Verification items for the finished model (mm, model axes). Coordinates: 2 decimals unless noted, no trailing zeros. Order: outer loops, then holes, each group sorted by start corner. A loop starts at its lowest first (then second) coordinate and runs counter-clockwise, first axis right, second up. Notation, with made-up numbers: (73, -9) -> (124, -9) arc R18 cw to (124, 25) -> close; hole circle Ø11 at (-34, -38). An arc over 180 degrees is marked (long way). Write each question's results on one line, items separated by ' | '. Start each with the question number.
(1) Cross-section at B-B on z = 5.5. Enter the section's corners in (x, y), and give its area (3 significant figures).
(2) Cross-section at C-C on x = 1.25. Enter the section's corners in (y, z), and give its area (3 significant figures).
(3) Cross-section at A-A on x = 4.75. Enter the section's corners in (y, z), and give its area (3 significant figures).
(4) Go/stop test with flat-tipped pins: pin 1 (12 mm diameter, centred on x = 9, z = 21, fed in from +Y); pin 2 (2 mm diameter, centred on x = 3, y = 7, fed in from -Z); pin 3 (2.5 mm diameter, centred on y = -2, z = 7.5, fed in from +X); pin 4 (1 mm diameter, centred on x = -9, z = 14.5, fed in from -Y). Record where each tip stops, or that it passes through.
(5) Thickness scan on probe 1 along X at (y, z) = (-4, 22.25); probe 2 along Y at (x, z) = (2.5, 23); probe 3 along X at (y, z) = (-3.25, 8). Record the ranges inside material, lowest first. Write a range as [from, to].
(6) Cross-section at D-D on y = -12. Enter the section's corners in (x, z).
(7) Draft check along Y on faces 1 (the flat face through (-0.2, -6.5, 0)), 2 (the flat face through (-4, 0, 12)). Enter one of: +Y half, -Y half, draft (parallel to the pull), parting line (faces both ways), or undercut.
```python
from build123d import *

# Parameters (mm, degrees)
BOSS_EXTRU_1_DEPTH = 25


with BuildPart() as part:
    # Esquisse2 → Boss.-Extru.1 (new body)
    with BuildSketch(Plane.XY):
        with BuildLine():
            ThreePointArc((-4, 4.472135955), (-2.140932539, 5.605034154), (0, 6))
            Line((0, 6), (0, 15))
            ThreePointArc((0, 15), (-2.018355219, 14.863587797), (-4, 14.456832295))
            Line((-4, 14.456832295), (-4, 4.472135955))
        make_face()
        with BuildLine():
            Line((0, 15), (0, 6))
            ThreePointArc((0, 6), (4.242640687, 4.242640687), (6, 0))
            ThreePointArc((6, 0), (2.449489743, -5.477225575), (-4, -4.472135955))
            Line((-4, -4.472135955), (-4, -14.456832295))
            ThreePointArc((-4, -14.456832295), (9.082951062, -11.937336386), (15, 0))
            ThreePointArc((15, 0), (10.606601718, 10.606601718), (0, 15))
        make_face()
        with BuildLine():
            ThreePointArc((-4, -4.472135955), (-6, 0), (-4, 4.472135955))
            Line((-4, 4.472135955), (-4, 14.456832295))
            ThreePointArc((-4, 14.456832295), (-15, 0), (-4, -14.456832295))
            Line((-4, -14.456832295), (-4, -4.472135955))
        make_face()
        with BuildLine():
            Line((-4, -4.472135955), (-4, 4.472135955))
            ThreePointArc((-4, 4.472135955), (-6, 0), (-4, -4.472135955))
        make_face()
    extrude(amount=BOSS_EXTRU_1_DEPTH)


solid = part.part
```
Results are:
1) outline: circle Ø30 at (0, 0); hole (-4, -4.47) arc R6 ccw (long way) to (-4, 4.47) -> close | area: 606 mm2
2) outline: (-14.95, 0) -> (-5.87, 0) -> (-5.87, 25) -> (-14.95, 25) -> close; (5.87, 0) -> (14.95, 0) -> (14.95, 25) -> (5.87, 25) -> close | area: 454 mm2
3) outline: (-14.23, 0) -> (-3.67, 0) -> (-3.67, 25) -> (-14.23, 25) -> close; (3.67, 0) -> (14.23, 0) -> (14.23, 25) -> (3.67, 25) -> close | area: 528 mm2
4) pin 1: stops at y = 14.7 | pin 2: stops at z = 0 | pin 3: stops at x = 14.98 | pin 4: stops at y = -12.36
5) probe 1: x = [-14.46, -4], [4.47, 14.46] | probe 2: y = [-14.79, -5.45], [5.45, 14.79] | probe 3: x = [-14.64, -4], [5.04, 14.64]
6) outline: (-9, 0) -> (9, 0) -> (9, 25) -> (-9, 25) -> close
7) face 1: draft | face 2: undercut
